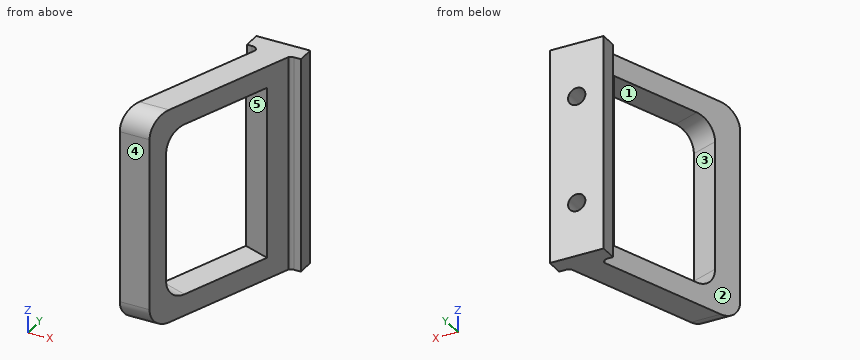
```python
from build123d import *

# Parameters (mm, degrees)
BOSS_EXTRUDE1_DEPTH       = 50
BOSS_EXTRUDE1_DEPTH_BACK  = 50
FILLET1_R                 = 10
CUT_EXTRUDE2_DEPTH        = 50
F_1_0MM_DOWEL_HOLE1_D     = 8
F_1_0MM_DOWEL_HOLE1_DEPTH = 15
F_1_0MM_DOWEL_HOLE1_TIP   = 2.403442476


with BuildPart() as part:
    # Sketch1 → Boss-Extrude1 (new body, two sides)
    with BuildSketch(Plane.XY) as boss_extrude1_sk:
        with BuildLine():
            Line((-12.5, 8), (12.5, 8))
            Line((12.5, 8), (12.5, 0))
            Line((12.5, 0), (9.375807417, 0))
            ThreePointArc((9.375807417, 0), (8.191786524, -0.243535865), (7.2, -0.93460365))
            Line((7.2, -0.93460365), (-18.665688958, -72))
            Line((-18.665688958, -72), (-32.5, -72))
            Line((-32.5, -72), (-7.2, -2.488821288))
            ThreePointArc((-7.2, -2.488821288), (-8.223971278, -0.705055977), (-10.156128604, 0))
            Line((-10.156128604, 0), (-12.5, 0))
            Line((-12.5, 0), (-12.5, 8))
        make_face()
    extrude(amount=BOSS_EXTRUDE1_DEPTH)
    extrude(boss_extrude1_sk.sketch, amount=-BOSS_EXTRUDE1_DEPTH_BACK)

    # Fillet1
    fillet1_edges = [part.edges().sort_by_distance(p)[0] for p in [
        (-25.582844479, -72, -50),
        (-25.582844479, -72, 50),
    ]]
    fillet(fillet1_edges, radius=FILLET1_R)

    # Sketch2 → Cut-Extrude2 (cut)
    with BuildSketch(Plane(origin=(-5.557868252, 2.02289861, 0), x_dir=(0, 0, 1), z_dir=(-0.939692621, 0.342020143, 0))):
        with BuildLine():
            Line((-40, -10.029869223), (40, -10.029869223))
            Line((40, -10.029869223), (40, -55.029869223))
            ThreePointArc((40, -55.029869223), (37.071067812, -62.100937034), (30, -65.029869223))
            Line((30, -65.029869223), (-30, -65.029869223))
            ThreePointArc((-30, -65.029869223), (-37.071067812, -62.100937034), (-40, -55.029869223))
            Line((-40, -55.029869223), (-40, -10.029869223))
        make_face()
    extrude(amount=-CUT_EXTRUDE2_DEPTH, mode=Mode.SUBTRACT)

    # 1.0mm Dowel Hole1
    with Locations(Plane(origin=(0, 8, 0), x_dir=(1, 0, 0), z_dir=(0, 1, 0))):
        with Locations((0, 25), (0, -25)):
            Hole(F_1_0MM_DOWEL_HOLE1_D / 2, depth=F_1_0MM_DOWEL_HOLE1_DEPTH)
            with Locations((0, 0, -(F_1_0MM_DOWEL_HOLE1_DEPTH + F_1_0MM_DOWEL_HOLE1_TIP / 2))):  # 118° drill point
                Cone(0, F_1_0MM_DOWEL_HOLE1_D / 2, F_1_0MM_DOWEL_HOLE1_TIP, mode=Mode.SUBTRACT)


solid = part.part
```
The listing builds one solid part. Answer for the finished solid, in the listing's coordinates (mm). Face numbers are marked on the shaded views. A direction names the side the tool comes from. Give positions to 0.01 mm unless a question says otherwise; leave off trailing zeros. Write each loop counter-clockwise with the first axis right and the second up, starting at its lowest first coordinate (ties: lowest second). Pieces come first, ordered by that corner, then holes. Notation, with made-up numbers: (2.5, 22) - (6.5, 22) arc R18 ccw to (6.5, 55) - close; hole circle Ø2 at (39.25, -36.5). An arc over 180 degrees is marked (long way). Use one line per item in the form item = value. Start each with the question number.
1) Find section C-C on z = -34.5. Determine the outline of the cut face in (x, y).
2) Find section B-B on y = -16.5. Determine the outline of the cut face in (x, z), plus the area to 3 significant figures.
3) Consider line 1 along Z through (x, y) = (0, -3.75); line 2 along X through (y, z) = (0.5, 25); line 3 along Y through (x, z) = (10, 14). Determine where each line is inside the solid, lowest interval first. Write a range as from..to.
4) Find section A-A on z = 9. Determine the outline of the cut face in (x, y).
5) A tool of negligible diameter and unlimited length cuts with its end or side. For the marked faces 4 and 5, from which of +Z, -Z, +X, -X, +Y, -Y can it reach the whole face along a straight path? Write none if from no direction.
6) Flat-ended cylindrical pins translate along their axes: pin 1 Ø0.9 at (x, z) = (10.5, 18.5) entering from -Y; pin 2 Ø5 at (x, z) = (0, -25) entering from -Y; pin 3 Ø4 at (y, z) = (2.5, 25) entering from -X. Find the tip coordinate at first contact, or state that the pin passes through.
7) The mould has two halves that part along Y. Classify the marked faces 1, 2 and 3: pulls with the +Y half, pulls with the -Y half, needs draft (parallel to the pull), parting line crosses it, or undercut.
Geometry results:
q1.outline = (-32.5, -72) - (-18.67, -72) - (-15.22, -62.53) - (-27.43, -58.08) - close; (-12.5, 0) - (-10.16, 0) arc R3 cw to (-7.2, -2.49) - (-8.99, -7.4) - (3.23, -11.85) - (7.2, -0.93) arc R3 cw to (9.38, 0) - (12.5, 0) - (12.5, 8) - (-12.5, 8) - close
q2.outline = (-12.3, -50) - (1.53, -50) - (1.53, -40) - (-12.3, -40) - close; (-12.3, 40) - (1.53, 40) - (1.53, 50) - (-12.3, 50) - close
q2.area = 277 mm2
q3.line_1 = -50..-29, -21..21, 29..50
q3.line_2 = -12.5..-4, 4..12.5
q3.line_3 = 0..8
q4.outline = (-32.5, -72) - (-18.67, -72) - (-15.58, -63.53) - (-27.8, -59.09) - close; (-12.5, 0) - (-10.16, 0) arc R3 cw to (-7.2, -2.49) - (-8.99, -7.4) - (3.23, -11.85) - (7.2, -0.93) arc R3 cw to (9.38, 0) - (12.5, 0) - (12.5, 8) - (-12.5, 8) - close
q5.face_4 = +Z, -Z, +X, -X, -Y
q5.face_5 = -X, -Y
q6.pin_1 = 0
q6.pin_2 = -11.58
q6.pin_3 = -12.5
q7.face_1 = needs draft
q7.face_2 = undercut
q7.face_3 = pulls with the +Y half
